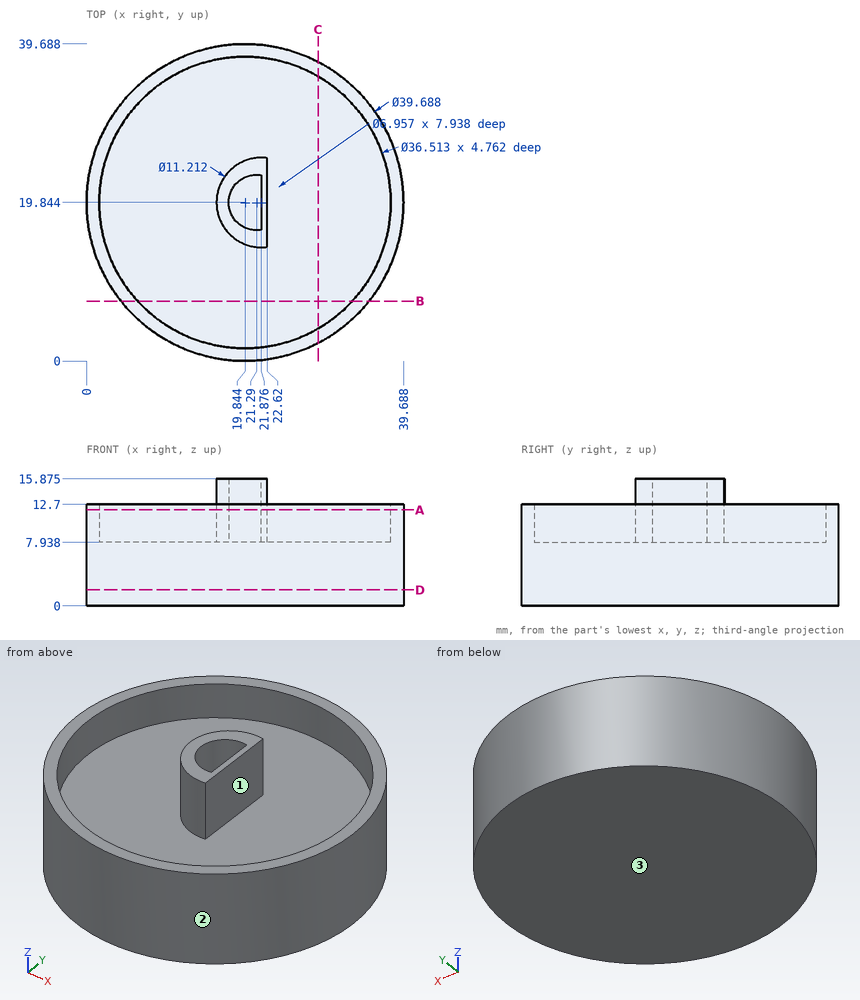
Geometry check sheet. Reference: drawing and pictorial views, mm from the part's lowest x, y, z. Round coordinates to 2 decimals unless told otherwise and drop trailing zeros. Loops run counter-clockwise (first coordinate to the right, second up) from the corner with the lowest first, then second, coordinate; pieces in that order, holes last. Notation, with made-up numbers: (52, 85.25) - (96, 85.25) arc R23 cw to (96, 99.25) - close; hole circle Ø9 at (27, -29.5). An arc over 180 degrees is marked (long way). Use a Markdown table: item, result.
Q1. Material ranges on line 1 (X direction, y = 17, z = 10) (1 decimal); line 2 (X direction, y = 22.5, z = 13.5) (1 decimal); line 3 (Z direction, x = 25, y = 34), recorded low to high.
Solutions:
| item | result |
|---|---|
| line 1 | x = 0.2 to 1.8, 17 to 19.3, 21.9 to 22.6, 37.9 to 39.5 |
| line 2 | x = 16.9 to 19, 21.9 to 22.6 |
| line 3 | z = 0 to 7.94 |
Q2. Cross-section at B-B on y = 7.5. Record the cut outline in (x, z) (1 decimal).
Solutions:
| item | result |
|---|---|
| outline | (4.3, 0) - (35.4, 0) - (35.4, 12.7) - (33.3, 12.7) - (33.3, 7.9) - (6.4, 7.9) - (6.4, 12.7) - (4.3, 12.7) - close |
Q3. Cross-section at A-A on z = 12. Record the cut outline in (x, y) (1 decimal).
Solutions:
| item | result |
|---|---|
| outline | circle Ø39.7 at (19.8, 19.8); (22.6, 14.3) - (22.6, 25.4) arc R5.6 ccw (long way) to start; hole circle Ø36.5 at (19.8, 19.8); hole (21.9, 16.4) - (21.9, 23.3) arc R3.5 ccw (long way) to start |
Q4. Cross-section at C-C on x = 29. Record the cut outline in (y, z).
Solutions:
| item | result |
|---|---|
| outline | (2.24, 0) - (37.45, 0) - (37.45, 12.7) - (35.64, 12.7) - (35.64, 7.94) - (4.05, 7.94) - (4.05, 12.7) - (2.24, 12.7) - close |
Q5. Go/stop test with flat-tipped pins: P1, Ø1.5, axis at y = 9, z = 4, coming from the -X side; P2, Ø1.5, axis at x = 18, z = 4.5, coming from the -Y side; P3, Ø1.5, axis at x = 15, z = 7.5, coming from the -Y side. Record where each tip stops, or that it passes through.
Solutions:
| item | result |
|---|---|
| P1 | stops at x = 2.76 |
| P2 | stops at y = 0.03 |
| P3 | stops at y = 0.43 |
Q6. Draft check along Y on the marked faces 1, 2 and 3. Enter one of: released by +Y, released by -Y, zero draft, split by the parting line, or undercut.
Solutions:
| item | result |
|---|---|
| face 1 | undercut |
| face 2 | split by the parting line |
| face 3 | zero draft |
Q7. Cross-section at D-D on z = 2. Record the cut outline in (x, y), plus the area to 3 significant figures.
Solutions:
| item | result |
|---|---|
| outline | circle Ø39.69 at (19.84, 19.84) |
| area | 1,240 mm2 |
